Design review of the part shown in the three views and the two pictorial views. Dimensions are in mm from the part's minimum x, y and z. A direction names the side the tool comes from. Give positions to 0.01 mm unless a question says otherwise; leave off trailing zeros. Write each loop counter-clockwise with the first axis right and the second up, starting at its lowest first coordinate (ties: lowest second). Pieces come first, ordered by that corner, then holes.
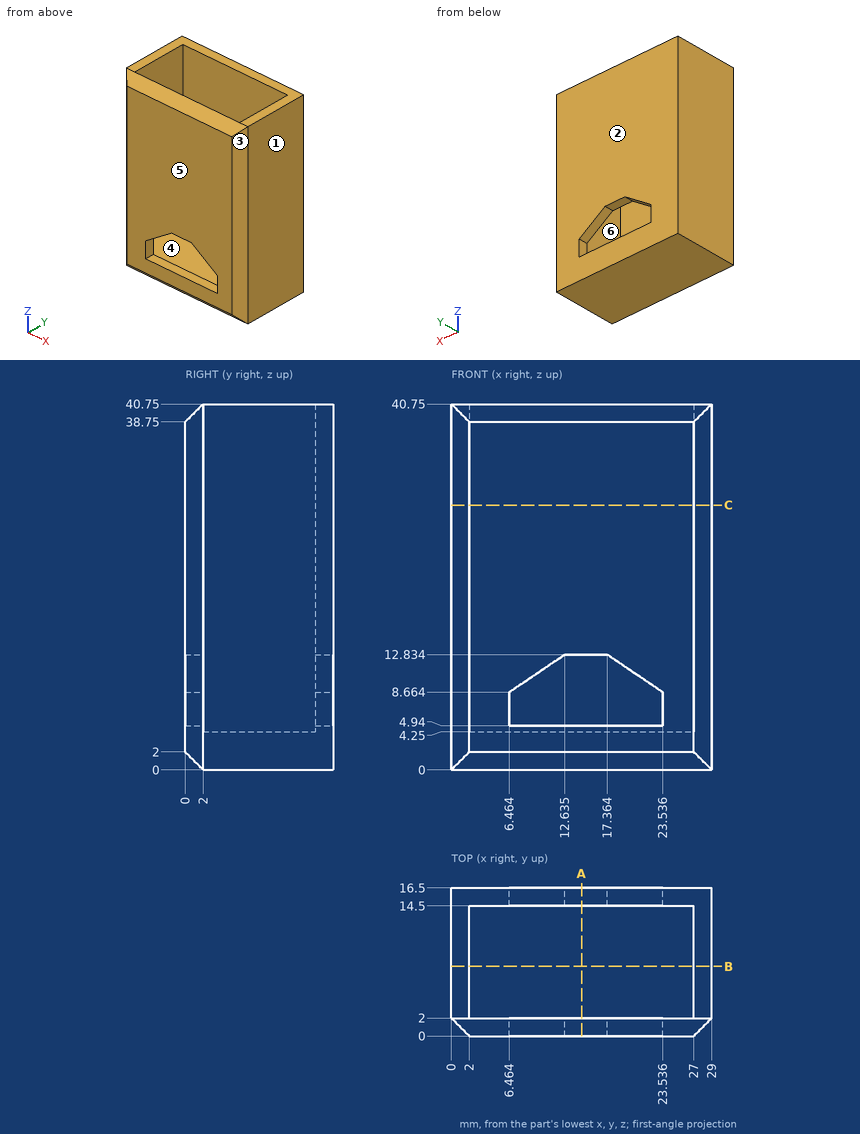
(1) Consider section B-B, the plane y = 7.75. Give the boundary of the cut face in (x, z), then the cut area to 3 significant figures.
Resolved:
outline: (0, 0) - (29, 0) - (29, 40.75) - (27, 40.75) - (27, 4.25) - (2, 4.25) - (2, 40.75) - (0, 40.75) - close
area: 269 mm2
(2) Consider section A-A, the plane x = 14.5. Give the number of separate pieces and of enclosed holes in the cut face, then the cut area to 3 significant figures.
Resolved:
separate pieces: 3
enclosed holes: 0
area: 181 mm2
(3) Consider section C-C, the plane z = 29.5. Give the boundary of the cut face in (x, y), then the cut area to 3 significant figures.
Resolved:
outline: (0, 2) - (2, 0) - (27, 0) - (29, 2) - (29, 16.5) - (0, 16.5) - close; hole (2, 2) - (27, 2) - (27, 14.5) - (2, 14.5) - close
area: 162 mm2
(4) Clearance check with flat-ended pins moving along their axes: P1, Ø1, axis at x = 14.5, y = 15.5, coming from the -Z side; P2, Ø2, axis at x = 19, y = 10.5, coming from the +Z side; P3, Ø1, axis at y = 1, z = 7.5, coming from the +X side; P4, Ø1, axis at x = 16, y = 1, coming from the -Z side. State where each tip first meets the part, or that it passes through.
Resolved:
P1: stops at z = 0
P2: stops at z = 4.25
P3: stops at x = 28.5
P4: stops at z = 0.5
(5) Mouldability with a two-part tool opening along Y and no side actions: class the marked faces 1, 2, 3 and 4 as pulls with the +Y half, pulls with the -Y half, needs draft (parallel to the pull), parting line crosses it, or undercut.
Resolved:
face 1: needs draft
face 2: pulls with the +Y half
face 3: pulls with the -Y half
face 4: undercut
(6) Tool access review of the marked faces 5 and 6: name each direction out of +Z, -Z, +X, -X, +Y, -Y from which nothing blocks a thin tool from reaching the whole face with its end or side.
Resolved:
face 5: +Z, -Z, +X, -X, -Y
face 6: +Z
(7) To check wall thickness, follow L1, parallel to Y at x = 20.25, z = 15.5; L2, parallel to X at y = 10.75, z = 29; L3, parallel to X at y = 15, z = 7.5. State the ranges of each line that lie inside material, in increasing order.
Resolved:
L1: y = 0 to 2, 14.5 to 16.5
L2: x = 0 to 2, 27 to 29
L3: x = 0 to 6.46, 23.54 to 29
